Geometry: see drawing. Coordinates: mm, zero at the bounding-box minimum. A direction names the side the tool comes from. Coordinates: 2 decimals unless noted, no trailing zeros. Write each loop counter-clockwise with the first axis right and the second up, starting at its lowest first coordinate (ties: lowest second). Pieces come first, ordered by that corner, then holes. Notation, with made-up numbers: (28.25, 65.25) - (75.25, 65.25) arc R16 cw to (75.25, 89.25) - close; hole circle Ø10 at (36, 18). An arc over 180 degrees is marked (long way). Use CSV: the item, a comma, the result in double quotes.
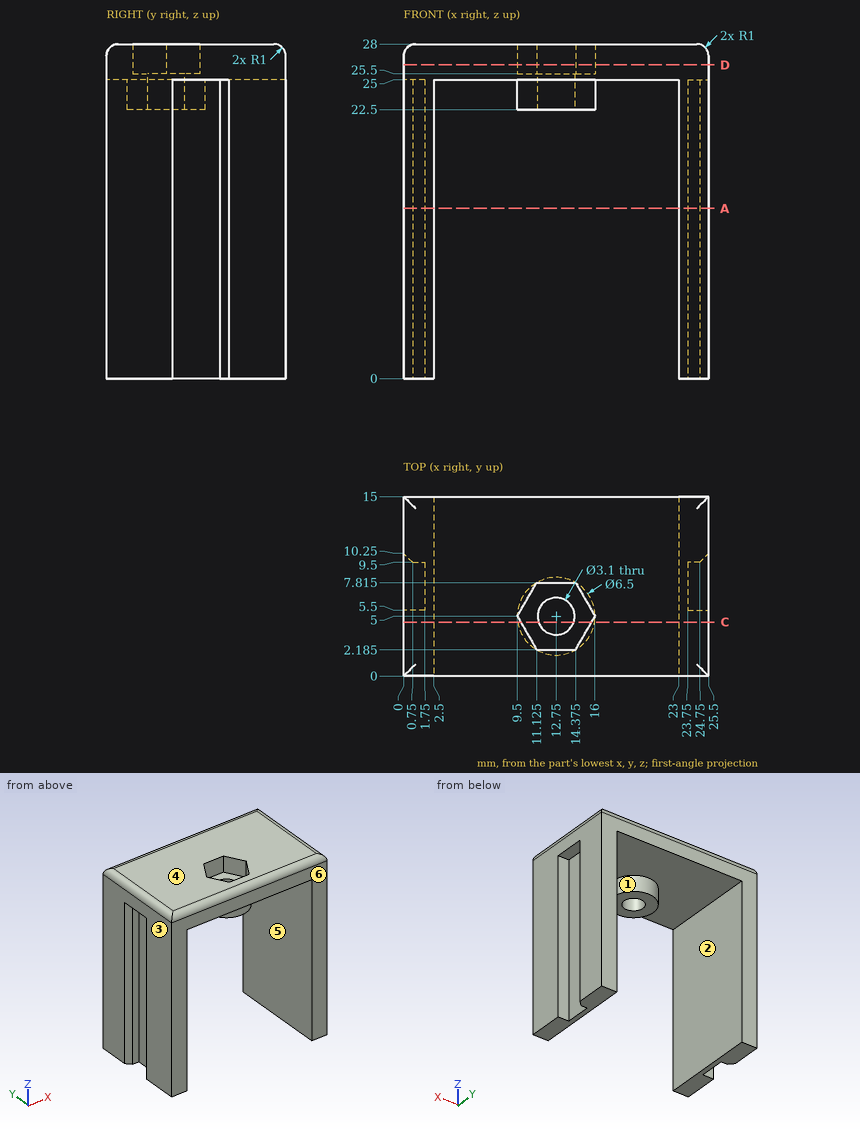
(1) Cut plane D-D on z = 26.25. Return loops of the section in (x, y) (1 decimal).
Check values:
outline,"(0, 0) - (25.5, 0) - (25.5, 15) - (0, 15) - close; hole (9.5, 5) - (11.1, 2.2) - (14.4, 2.2) - (16, 5) - (14.4, 7.8) - (11.1, 7.8) - close"
(2) Pin query (flat end, axial travel): pin 1 Ø1.4 at (x, y) = (1, 8) entering from -Z; pin 2 Ø2 at (y, z) = (7, 5) entering from +X; pin 3 Ø3.5 at (x, y) = (12.75, 5) entering from -Z. Return the tip coordinate at first contact, or that it passes through.
Check values:
pin 1,"z = 25"
pin 2,"x = 23.75"
pin 3,"z = 22.5"
(3) Reachability of the marked faces 5 and 6 from +Z, -Z, +X, -X, +Y, -Y: full face, straight path, thin tool, end or side. Return the list, or none.
Check values:
face 5,"-Z, +Y, -Y"
face 6,"+Z, -Z, +X, -X, -Y"
(4) Cut plane A-A on z = 14.25. Return loops of the section in (x, y).
Check values:
outline,"(0, 0) - (2.5, 0) - (2.5, 15) - (0, 15) - (0, 10.25) - (0.75, 9.5) - (1.75, 9.5) - (1.75, 5.5) - (0, 5.5) - close; (23, 0) - (25.5, 0) - (25.5, 5.5) - (23.75, 5.5) - (23.75, 9.5) - (24.75, 9.5) - (25.5, 10.25) - (25.5, 15) - (23, 15) - close"
(5) Ray query, probe 1 along Y at (x, z) = (12.75, 23.4); probe 2 along X at (y, z) = (12.25, 24.5); probe 3 along X at (y, z) = (7.25, 21.5). Return the intervals inside material, ascending. Write a range as from..to.
Check values:
probe 1,"1.75..3.45, 6.55..8.25"
probe 2,"0..2.5, 23..25.5"
probe 3,"1.75..2.5, 23..23.75"
(6) Cut plane C-C on y = 4.5. Return loops of the section in (x, z).
Check values:
outline,"(0, 0) - (2.5, 0) - (2.5, 25) - (9.54, 25) - (9.54, 22.5) - (11.28, 22.5) - (11.28, 25.5) - (9.79, 25.5) - (9.79, 28) - (1, 28) arc R1 ccw to (0, 27) - close; (14.22, 22.5) - (15.96, 22.5) - (15.96, 25) - (23, 25) - (23, 0) - (25.5, 0) - (25.5, 27) arc R1 ccw to (24.5, 28) - (15.71, 28) - (15.71, 25.5) - (14.22, 25.5) - close"
(7) Draft query along X for the marked faces 1, 2, 3 and 4. Return one class per face: pulls with the +X half, pulls with the -X half, needs draft (parallel to the pull), parting line crosses it, or undercut.
Check values:
face 1,"undercut"
face 2,"undercut"
face 3,"pulls with the -X half"
face 4,"needs draft"
